Check sheet for the drawn part. Datum: minimum x, y, z corner. Units: mm. Coordinates: 2 decimals unless noted, no trailing zeros. Order: outer loops, then holes, each group sorted by start corner. A loop starts at its lowest first (then second) coordinate and runs counter-clockwise, first axis right, second up.
Q1. Cross-section at A-A, the plane y = 22.5. Record the boundary of the cut face in (x, z).
Q2. Cross-section at B-B, the plane z = 1.35. Record the boundary of the cut face in (x, y).
Q3. Cross-section at C-C, the plane x = 21.5. Record the boundary of the cut face in (y, z), and give its area (3 significant figures).
Q4. Thickness scan on line 1 (Y direction, x = 9.8, z = 0.95); line 2 (Y direction, x = 21.5, z = 0.95). Record the ranges inside material, lowest first.
Q5. Cross-section at D-D, the plane x = 9.8. Record the boundary of the cut face in (y, z).
Q6. Depth check by flat-ended pin: P1, Ø0.6, axis at y = 23, z = 0.5, coming from the +X side; P2, Ø1, axis at x = 11.5, z = 1.5, coming from the -Y side; P3, Ø3.5, axis at x = 9.8, y = 35.2, coming from the +Z side; P4, Ø1, axis at y = 5, z = 1, coming from the +X side. Enter the tip coordinate at first touch or a pass-through.
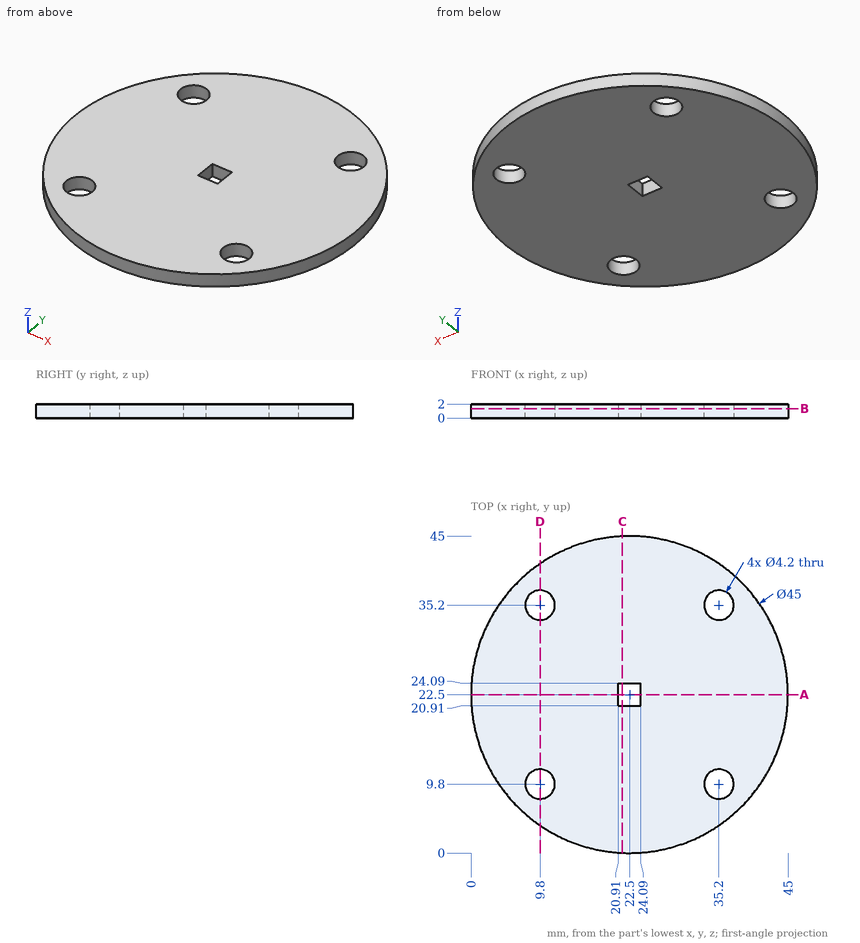
Check values:
1. outline: (0, 0) - (20.91, 0) - (20.91, 2) - (0, 2) - close; (24.09, 0) - (45, 0) - (45, 2) - (24.09, 2) - close
2. outline: circle Ø45 at (22.5, 22.5); hole circle Ø4.2 at (9.8, 9.8); hole circle Ø4.2 at (9.8, 35.2); hole (20.91, 20.91) - (24.09, 20.91) - (24.09, 24.09) - (20.91, 24.09) - close; hole circle Ø4.2 at (35.2, 9.8); hole circle Ø4.2 at (35.2, 35.2)
3. outline: (0.02, 0) - (20.91, 0) - (20.91, 2) - (0.02, 2) - close; (24.09, 0) - (44.98, 0) - (44.98, 2) - (24.09, 2) - close
3. area: 83.6 mm2
4. line 1: y = 3.93 to 7.7, 11.9 to 33.1, 37.3 to 41.07
4. line 2: y = 0.02 to 20.91, 24.09 to 44.98
5. outline: (3.93, 0) - (7.7, 0) - (7.7, 2) - (3.93, 2) - close; (11.9, 0) - (33.1, 0) - (33.1, 2) - (11.9, 2) - close; (37.3, 0) - (41.07, 0) - (41.07, 2) - (37.3, 2) - close
6. P1: stops at x = 45
6. P2: stops at y = 2.6
6. P3: passes through
6. P4: stops at x = 37.24
